```python
from build123d import *

# Parameters (mm, degrees)
F0_R     = 9.525
F1_DEPTH = 44.45
F3_DEPTH = 12.7
F4_R     = 6.35


with BuildPart() as f1:
    # F0 (on Top) → F1 (new body)
    with BuildSketch(Plane.XY):
        with BuildLine():
            ThreePointArc((0, 19.960436), (11.258275, 16.482422), (18.593146, 7.260436))
            Line((18.593146, 7.260436), (88.9, 7.260436))
            Line((88.9, 7.260436), (88.9, 19.960436))
            Line((88.9, 19.960436), (0, 19.960436))
        make_face()
        with BuildLine():
            ThreePointArc((0, 19.960436), (-14.114159, -14.114159), (19.960436, 0))
            ThreePointArc((19.960436, 0), (19.615635, 3.694029), (18.593146, 7.260436))
            ThreePointArc((18.593146, 7.260436), (11.258275, 16.482422), (0, 19.960436))
        make_face()
        Circle(F0_R, mode=Mode.SUBTRACT)
    extrude(amount=F1_DEPTH)

    # F2 (on face) → F3 (cut)
    with BuildSketch(Plane.XZ.offset(-7.260436)):
        with BuildLine():
            Line((88.9, 14.2748), (88.9, 30.1498))
            Line((88.9, 30.1498), (38.1, 30.1498))
            ThreePointArc((38.1, 30.1498), (43.71266, 27.82496), (46.0375, 22.2123))
            ThreePointArc((46.0375, 22.2123), (43.71266, 16.59964), (38.1, 14.2748))
            Line((38.1, 14.2748), (88.9, 14.2748))
        make_face()
        with BuildLine():
            Line((38.1, 14.2748), (38.1, 30.1498))
            ThreePointArc((38.1, 30.1498), (30.1625, 22.2123), (38.1, 14.2748))
        make_face()
        with BuildLine():
            ThreePointArc((46.0375, 22.2123), (43.71266, 27.82496), (38.1, 30.1498))
            Line((38.1, 30.1498), (38.1, 14.2748))
            ThreePointArc((38.1, 14.2748), (43.71266, 16.59964), (46.0375, 22.2123))
        make_face()
    extrude(amount=-F3_DEPTH, mode=Mode.SUBTRACT)

    # F4
    f4_edges = [f1.edges().sort_by_distance(p)[0] for p in [
        (18.593146, 7.260436, 22.225),
    ]]
    fillet(f4_edges, radius=F4_R)


solid = f1.part
```
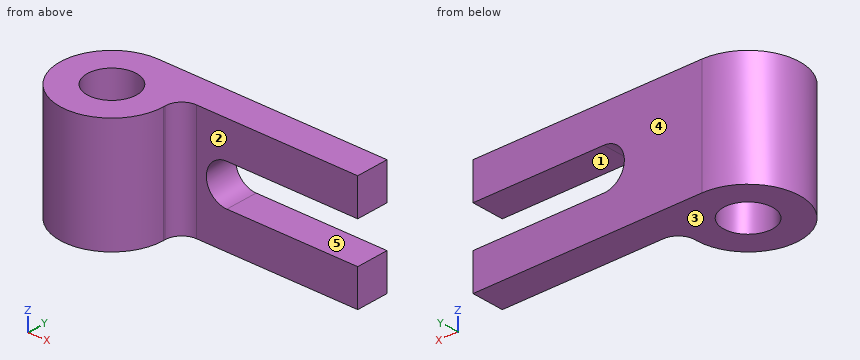
Source: CAD feature listing. Evaluate the final solid. Frame: model axes, mm. Face numbers are marked on the shaded views. A direction names the side the tool comes from. Round coordinates to 2 decimals unless told otherwise and drop trailing zeros. Order: outer loops, then holes, each group sorted by start corner. A loop starts at its lowest first (then second) coordinate and runs counter-clockwise, first axis right, second up. Notation, with made-up numbers: (67.25, -5.5) -> (79.25, -5.5) arc R19 cw to (79.25, 13.5) -> close; hole circle Ø11 at (-5, 37.25). An arc over 180 degrees is marked (long way). One line per item, written item: value. Start each with the question number.
Q1. Section query C-C (y = -4). Return the cut outline in (x, z), plus the area to 3 significant figures.
Q2. Draft query along Z for the marked faces 1, 2 and 3. Return one class per face: pulls with the +Z half, pulls with the -Z half, needs draft (parallel to the pull), parting line crosses it, or undercut.
Q3. Section query D-D (z = 23). Return the cut outline in (x, y) (3 decimals).
Q4. Pin query (flat end, axial travel): pin 1 (5 mm diameter, centred on x = -7, z = 9, fed in from +Y); pin 2 (15 mm diameter, centred on x = 0, y = 0, fed in from -Z); pin 3 (6.5 mm diameter, centred on x = 63.5, y = 13.5, fed in from -Z); pin 4 (1 mm diameter, centred on y = 11.5, z = 15.5, fed in from +X). Return the tip coordinate at first contact, or that it passes through.
Q5. Section query B-B (z = 40.5). Return the cut outline in (x, y) (3 decimals), plus the area to 3 significant figures.
Q6. Access query for the marked faces 4 and 5. Directions: +Z, -Z, +X, -X, +Y, -Y. A direction counts if a zero-diameter tool reaches every point of the face in a straight line with its end or side. Return the directions, or none.
Q7. Section query A-A (x = 40.5). Return the cut outline in (y, z), plus the area to 3 significant figures.
Q8. Material intervals for probe 1 along Y at (x, z) = (53, 40.5); probe 2 along Z at (x, y) = (40.5, 9.5); probe 3 along X at (y, z) = (-1, 34.5), sorted ascending.
Findings below:
1. outline: (-19.56, 0) -> (-8.64, 0) -> (-8.64, 44.45) -> (-19.56, 44.45) -> close; (8.64, 0) -> (19.56, 0) -> (19.56, 44.45) -> (8.64, 44.45) -> close
1. area: 970 mm²
2. face 1: undercut
2. face 2: needs draft
2. face 3: pulls with the -Z half
3. outline: (0, 19.96) arc R19.96 ccw (long way) to (19.96, 0) arc R19.96 ccw to (19.948, 0.691) arc R6.35 cw to (26.295, 7.26) -> (30.202, 7.26) -> (30.202, 19.96) -> close; hole circle Ø19.05 at (0, 0)
4. pin 1: y = 19.45
4. pin 2: through
4. pin 3: z = 0
4. pin 4: x = 34.79
5. outline: (0, 19.96) arc R19.96 ccw (long way) to (19.96, 0) arc R19.96 ccw to (19.948, 0.691) arc R6.35 cw to (26.295, 7.26) -> (88.9, 7.26) -> (88.9, 19.96) -> close; hole circle Ø19.05 at (0, 0)
5. area: 1,940 mm²
6. face 4: +Z, -Z, +X, -X, +Y
6. face 5: +X, +Y, -Y
7. outline: (7.26, 0) -> (19.96, 0) -> (19.96, 14.27) -> (7.26, 14.27) -> close; (7.26, 30.15) -> (19.96, 30.15) -> (19.96, 44.45) -> (7.26, 44.45) -> close
7. area: 363 mm²
8. probe 1: 7.26 to 19.96
8. probe 2: 0 to 14.27, 30.15 to 44.45
8. probe 3: -19.94 to -9.47, 9.47 to 19.94
